Autodesk Fusion 360 part; units mm, degrees
sketch "Sketch1" plane through (0, 0, 0) normal (0, 1, 0) x (1, 0, 0)
  line L0 (0, 0) -> (20, 0)
  line L1 (20, 0) -> (20, -12.8)
  line L2 (20, -12.8) -> (0, -12.8)
  line L3 (0, -12.8) -> (0, 0)
  dimension "d1" = 20
  dimension "d2" = 12.8
extrude "Extrude1" add sketch "Sketch1" along normal blind 10
sketch "Sketch2" plane through (0, 10, 0) normal (0, 1, 0) x (-1, 0, 0)
  line L0 (0, 12.8) -> (-20, 12.8)
  line L1 (-20, 12.8) -> (-20, 0)
  line L2 (-20, 0) -> (0, 0)
  line L3 (0, 0) -> (0, 12.8)
  line L4 (-10, 0) -> (-10, 12.8) construction
  line L5 (0, 6.4) -> (-20, 6.4) construction
  point P0 (-10, 6.4)
hole "Hole1" at (10, 10, 6.4) direction (0, -1, 0) diameter 2.5 end through all
sketch "Sketch3" plane through (0, 0, 12.8) normal (0, 0, 1) x (1, 0, 0)
  line L0 (0, 0) -> (20, 0)
  line L1 (20, 0) -> (20, 10)
  line L2 (20, 10) -> (0, 10)
  line L3 (0, 10) -> (0, 0)
  line L4 (0, 5) -> (20, 5) construction
  line L5 (5, 2.6) -> (5, 7.2) construction
  line L6 (15, 2.6) -> (15, 7.2) construction
  point P0 (5, 5)
  point P1 (15, 5)
  dimension "d8" = 10
  dimension "d9" = 5
  dimension "d16" = 5
hole "Hole4" at (5, 5, 12.8) direction (0, 0, -1) diameter 2.5 end through all
hole "Hole5" at (15, 5, 12.8) direction (0, 0, -1) diameter 2.5 end through all
Input: part model. Units: mm. Frame: model coordinates. Give positions to 0.01 mm unless a question says otherwise; leave off trailing zeros. Order: outer loops, then holes, each group sorted by start corner. A loop starts at its lowest first (then second) coordinate and runs counter-clockwise, first axis right, second up. Notation, with made-up numbers: M 71,24.5 L 89,24.5 A20 cw 89,43.5 Z; hole C 68.25,40 d4. An arc over 180 degrees is marked long. One line per question, with ' | ' between items.
1) Section D-D on z = 8. Output: boundary loops of the cut face in (x, y), and give its area (3 significant figures).
Filled in:
outline: M 0,0 L 20,0 L 20,10 L 0,10 Z; hole C 5,5 d2.5; hole C 15,5 d2.5 | area: 190 mm2
2) Ray query, L1, parallel to X at y = 5, z = 8; L2, parallel to Y at x = 15, z = 5.5; L3, parallel to Z at x = 10, y = 3.75. Return the intervals inside material, ascending.
Filled in:
L1: x = 0 to 3.75, 6.25 to 13.75, 16.25 to 20 | L2: y = 0 to 3.75, 6.25 to 10 | L3: z = 0 to 5.15, 7.65 to 12.8
3) Section A-A on x = 5.75. Output: boundary loops of the cut face in (y, z), and give its area (3 significant figures).
Filled in:
outline: M 0,0 L 4,0 L 4,12.8 L 0,12.8 Z; M 6,0 L 10,0 L 10,12.8 L 6,12.8 Z | area: 102 mm2
4) Draft query along X for faces 1 (the face through (6.22, 5.27, 6.31)), 2 (the face through (0, 5, 6)), 3 (the face through (8.76, 4.93, 6.24)), 4 (the face through (10, 10, 8)). Return one class per face: pulls with the +X half, pulls with the -X half, needs draft (parallel to the pull), parting line crosses it, or undercut.
Filled in:
face 1: undercut | face 2: pulls with the -X half | face 3: undercut | face 4: needs draft
5) Contact query for a flat-ended pin moving along its axis: P1, Ø1.5, axis at x = 7.5, z = 6, coming from the -Y side. Output: stop coordinate, or through.
Filled in:
P1: stops at y = 0
6) Section C-C on y = 5. Output: boundary loops of the cut face in (x, z), and give its area (3 significant figures).
Filled in:
outline: M 0,0 L 3.75,0 L 3.75,12.8 L 0,12.8 Z; M 6.25,0 L 13.75,0 L 13.75,12.8 L 6.25,12.8 Z; M 16.25,0 L 20,0 L 20,12.8 L 16.25,12.8 Z; hole C 10,6.4 d2.5 | area: 187 mm2
7) Section B-B on z = 6.4. Output: boundary loops of the cut face in (x, y).
Filled in:
outline: M 0,0 L 8.75,0 L 8.75,10 L 0,10 Z; M 11.25,0 L 20,0 L 20,10 L 11.25,10 Z; hole C 5,5 d2.5; hole C 15,5 d2.5
